```python
from build123d import *

# Parameters (mm, degrees)
SKETCH1_R               = 32
SKETCH1_R_2             = 3
BOSS_EXTRUDE1_DEPTH     = 10
SKETCH2_R               = 15
SKETCH2_R_2             = 10.25
BOSS_EXTRUDE2_DEPTH     = 37
SKETCH3_R               = 3
CUT_EXTRUDE1_DEPTH      = 33
CUT_EXTRUDE1_DEPTH_BACK = 33
FILLET_1_R              = 5
CHAMFER_1_SIZE          = 1


with BuildPart() as part:
    # Sketch1 → Boss-Extrude1 (new body)
    with BuildSketch(Plane.XY):
        Circle(SKETCH1_R)
        with Locations((20, 11.547005384)):
            Circle(SKETCH1_R_2, mode=Mode.SUBTRACT)
        with Locations((0, -23.094010768)):
            Circle(SKETCH1_R_2, mode=Mode.SUBTRACT)
        with Locations((-20, 11.547005384)):
            Circle(SKETCH1_R_2, mode=Mode.SUBTRACT)
    extrude(amount=BOSS_EXTRUDE1_DEPTH)

    # Sketch2 → Boss-Extrude2 (add)
    with BuildSketch(Plane.XY.offset(10)):
        Circle(SKETCH2_R)
        Circle(SKETCH2_R_2, mode=Mode.SUBTRACT)
    extrude(amount=BOSS_EXTRUDE2_DEPTH)

    # Sketch3 → Cut-Extrude1 (cut, two sides)
    with BuildSketch(Plane(origin=(0, 0, 0), x_dir=(1, 0, 0), z_dir=(0, 1, 0))) as cut_extrude1_sk:
        with Locations((0, -30)):
            Circle(SKETCH3_R)
    extrude(amount=CUT_EXTRUDE1_DEPTH, mode=Mode.SUBTRACT)
    extrude(cut_extrude1_sk.sketch, amount=-CUT_EXTRUDE1_DEPTH_BACK, mode=Mode.SUBTRACT)

    # 圆角1
    fillet_1_edges = [part.edges().sort_by_distance(p)[0] for p in [
        (-15, 0, 10),
    ]]
    fillet(fillet_1_edges, radius=FILLET_1_R)

    # 倒角1
    chamfer_1_edges = [part.edges().sort_by_distance(p)[0] for p in [
        (-15, 0, 47),
        (-32, 0, 10),
    ]]
    chamfer(chamfer_1_edges, length=CHAMFER_1_SIZE)


solid = part.part
```
Could you check a few things on this model? Use its own coordinates, in mm. A direction names the side the tool comes from. Round coordinates to 2 decimals unless told otherwise and drop trailing zeros. Loops run counter-clockwise (first coordinate to the right, second up) from the corner with the lowest first, then second, coordinate; pieces in that order, holes last.
Q1. Please list where these lines run through material, in increasing order: L1, parallel to Z at x = 0, y = 12; L2, parallel to Y at x = 0, z = 7.5; L3, parallel to X at y = -24, z = 2.
Q2. I want a section at B-B (z = 30). Write out the boundary of the cut face in (x, y).
Q3. I want a section at A-A (x = 0). Give the number of separate pieces and of enclosed holes in the cut face, and give its area (3 significant figures).
Q4. Thinking about a two-plate mould opening in X: for faces 3 (the cylindrical face through (17.003, 11.679, 4.93)), 4 (the cylindrical face through (-3.252, -14.643, 30.283)), 5 (the flat face through (-1.1, 10.4, 47)), which applies, pulls with the +X half, pulls with the -X half, needs draft (parallel to the pull), parting line crosses it, or undercut?
Q5. On a 3-axis mill with a long thin cutter (end or side, diameter ignored), from which of +Z, -Z, +X, -X, +Y, -Y can I reach the whole of each face in a straight line? I mean faces 1 (the flat face through (0, 0, 10)), 2 (the cylindrical face through (-6.94, -31.24, 4.44)). Say none if no direction works.
Q6. I want a section at D-D (z = 16). Write out the boundary of the cut face in (x, y), and give its area (3 significant figures).
Q7. For P1, Ø5, axis at y = -8.5, z = 15, coming from the +X side; P2, Ø2, axis at x = -10, z = 20, coming from the -Y side; P3, Ø5, axis at x = -20, y = 11.55, coming from the -Z side; P4, Ø7, axis at x = 0, y = -23.09, coming from the +Z side, each with a flat end and sliding along its axis, tell me the tip position at first contact or that it passes through.
Q8. I want a section at C-C (y = 0). Write out the boundary of the cut face in (x, z).
Answer below:
1. L1: z = 0 to 27, 33 to 47
1. L2: y = -32 to -26.09, -20.09 to 32
1. L3: x = -21.17 to -2.86, 2.86 to 21.17
2. outline: (-3, -14.7) - (-3, -9.8) arc R10.25 cw to (-3, 9.8) - (-3, 14.7) arc R15 ccw to start; (3, -14.7) arc R15 ccw to (3, 14.7) - (3, 9.8) arc R10.25 cw to (3, -9.8) - close
3. separate pieces: 4
3. enclosed holes: 0
3. area: 883 mm2
4. face 3: undercut
4. face 4: parting line crosses it
4. face 5: needs draft
5. face 1: +Z
5. face 2: +Z, -Z
6. outline: circle Ø30 at (0, 0); hole circle Ø20.5 at (0, 0)
6. area: 377 mm2
7. P1: stops at x = 13.77
7. P2: stops at y = -12
7. P3: passes through
7. P4: stops at z = 10.02
8. outline: (-32, 0) - (32, 0) - (32, 9) - (31, 10) - (20, 10) arc R5 cw to (15, 15) - (15, 46) - (14, 47) - (10.25, 47) - (10.25, 10) - (-10.25, 10) - (-10.25, 47) - (-14, 47) - (-15, 46) - (-15, 15) arc R5 cw to (-20, 10) - (-31, 10) - (-32, 9) - close
